Check sheet for the drawn part. Datum: minimum x, y, z corner. Units: mm. A direction names the side the tool comes from. Coordinates: 2 decimals unless noted, no trailing zeros. Write each loop counter-clockwise with the first axis right and the second up, starting at its lowest first coordinate (ties: lowest second). Pieces come first, ordered by that corner, then holes. Notation, with made-up numbers: (3.25, 39) -> (56.25, 39) arc R10 cw to (56.25, 49) -> close; hole circle Ø10 at (-0.5, 72). An arc over 180 degrees is marked (long way). Answer in a Markdown table with one row per item. Add a question column.
Q1. Tool access check on the marked faces 1 and 2. Record the directions out of +Z, -Z, +X, -X, +Y, -Y that give a thin tool (end or side, any length) a straight path to the whole face; none if there is none.
Q2. Thickness scan on line 1 (Z direction, x = 3.5, y = 39.5); line 2 (Y direction, x = 6.5, z = 3.25). Record the ranges inside material, lowest first.
Q3. Section check D-D, the plane x = 0.5. Record the boundary of the cut face in (y, z).
Q4. Section check B-B, the plane x = 3.5. Record the boundary of the cut face in (y, z), and give its area (3 significant figures).
Q5. Section check C-C, the plane y = 9.5. Record the boundary of the cut face in (x, z), and give its area (3 significant figures).
Q6. Gauge pin test, flat ends, axial feed: P1, Ø2, axis at x = 3, y = 36, coming from the +Z side; P2, Ø1.5, axis at x = 5.5, z = 6.5, coming from the +Y side; P3, Ø2, axis at x = 4.5, y = 25, coming from the -Z side; P4, Ø2, axis at x = 6, z = 2, coming from the +Y side. Record the tip position at first contact, or that the pin passes through.
Q7. Section check A-A, the plane z = 3.5. Record the boundary of the cut face in (x, y).
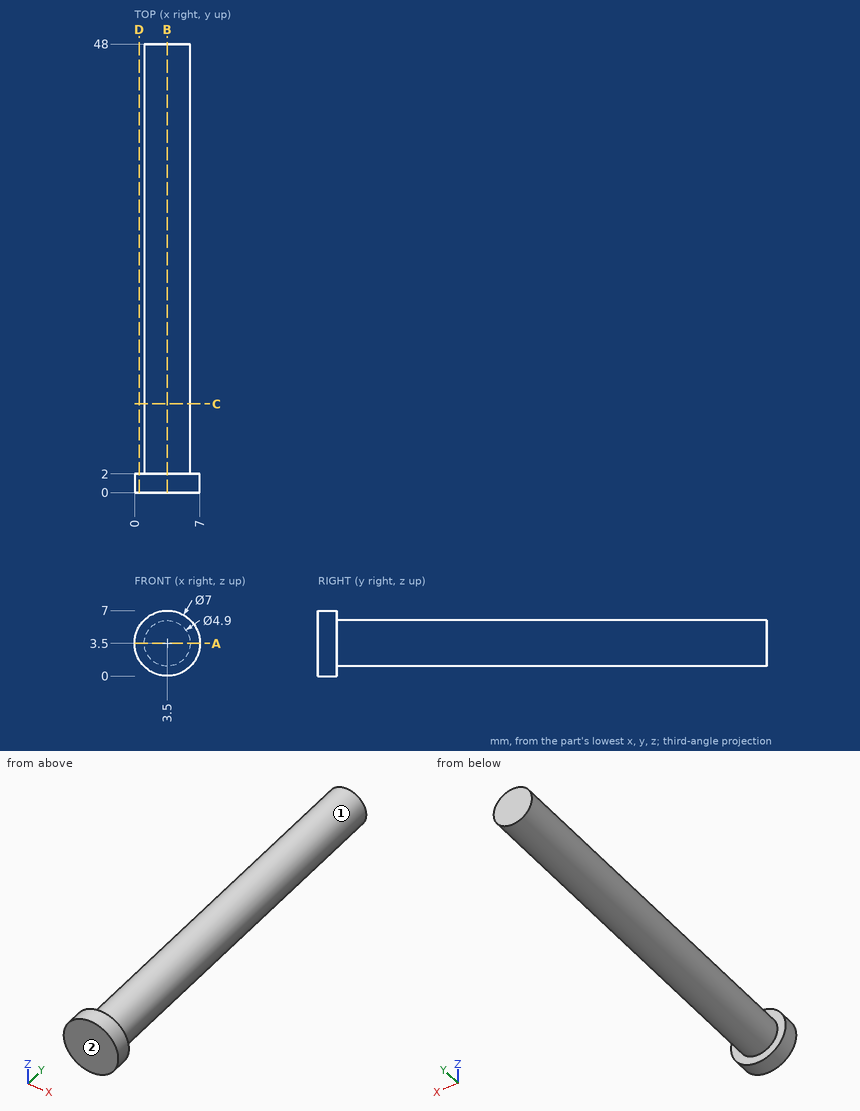
Calculated:
| question | item | result |
|---|---|---|
| 1 | face 1 | +Y |
| 1 | face 2 | +Z, -Z, +X, -X, -Y |
| 2 | line 1 | z = 1.05 to 5.95 |
| 2 | line 2 | y = 0 to 2 |
| 3 | outline | (0, 1.7) -> (2, 1.7) -> (2, 5.3) -> (0, 5.3) -> close |
| 4 | outline | (0, 0) -> (2, 0) -> (2, 1.05) -> (48, 1.05) -> (48, 5.95) -> (2, 5.95) -> (2, 7) -> (0, 7) -> close |
| 4 | area | 239 mm² |
| 5 | outline | circle Ø4.9 at (3.5, 3.5) |
| 5 | area | 18.9 mm² |
| 6 | P1 | stops at z = 5.95 |
| 6 | P2 | stops at y = 2 |
| 6 | P3 | stops at z = 1.05 |
| 6 | P4 | stops at y = 48 |
| 7 | outline | (0, 0) -> (7, 0) -> (7, 2) -> (5.95, 2) -> (5.95, 48) -> (1.05, 48) -> (1.05, 2) -> (0, 2) -> close |
